For this review, take the finished solid that the model builds, in its own axes (mm). Round coordinates to 2 decimals unless told otherwise and drop trailing zeros. Order: outer loops, then holes, each group sorted by start corner. A loop starts at its lowest first (then second) coordinate and runs counter-clockwise, first axis right, second up. Notation, with made-up numbers: (-6, 69) -> (8, 69) arc R10 cw to (8, 82) -> close; hole circle Ø4 at (-24.75, -28). An arc over 180 degrees is marked (long way). Use a Markdown table: item, result. Add a question column.
1) Consider section B-B (y = 93). State the section outline as (x, z) points (1 decimal).
2) Clearance check with flat-ended pins moving along their axes: P1, Ø10, axis at x = -6, y = 41.5, coming from the -Z side; P2, Ø1.5, axis at x = 0, y = 47.5, coming from the -Z side; P3, Ø1.9, axis at x = 0.5, z = -11, coming from the +Y side. State where each tip first meets the part, or that it passes through.
3) Wall thickness on line 1 along Y through (x, z) = (-1, -10); line 2 along X through (y, z) = (31.5, -0.25): over which ranges is each line inside the solid? List them lowest first. Write a range as [from, to].
4) Consider section C-C (y = 59). State the section outline as (x, z) points.
5) Consider section A-A (x = 0). State the section outline as (y, z) points.
6) Consider section D-D (z = -3.25). State the section outline as (x, y) points, plus the area to 3 significant figures.
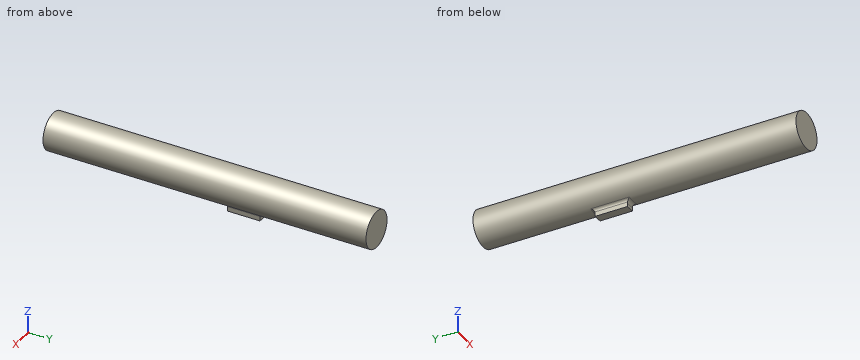
```python
from build123d import *

# Parameters (mm, degrees)
SKETCH1_R           = 8.5
BOSS_EXTRUDE1_DEPTH = 150
SKETCH5_W           = 4
SKETCH5_H           = 11.5
BOSS_EXTRUDE2_DEPTH = 15
FILLET1_R           = 1.5


with BuildPart() as part:
    # Sketch1 → Boss-Extrude1 (new body)
    with BuildSketch(Plane(origin=(0, 0, 0), x_dir=(1, 0, 0), z_dir=(0, 1, 0))):
        Circle(SKETCH1_R)
    extrude(amount=BOSS_EXTRUDE1_DEPTH)

    # Sketch5 → Boss-Extrude2 (add)
    with BuildSketch(Plane(origin=(0, 82.02, 0), x_dir=(1, 0, 0), z_dir=(0, 1, 0))):
        with Locations((0, 5.75)):
            Rectangle(SKETCH5_W, SKETCH5_H)
    extrude(amount=BOSS_EXTRUDE2_DEPTH)

    # Fillet1
    fillet1_edges = [part.edges().sort_by_distance(p)[0] for p in [
        (0, 82.02, -8.5),
        (-2, 89.52, -8.261355821),
        (2, 89.52, -8.261355821),
        (0, 97.02, -8.5),
    ]]
    fillet(fillet1_edges, radius=FILLET1_R)


solid = part.part
```
Results list:
| question | item | result |
|---|---|---|
| 1 | outline | (-3, -8) arc R1.5 cw to (-2, -9.4) -> (-2, -11.5) -> (2, -11.5) -> (2, -9.4) arc R1.5 cw to (3, -8) arc R8.5 ccw (long way) to start |
| 2 | P1 | z = -8.44 |
| 2 | P2 | z = -8.5 |
| 2 | P3 | y = 97.02 |
| 3 | line 1 | [82.02, 97.02] |
| 3 | line 2 | [-8.5, 8.5] |
| 4 | outline | circle Ø17 at (0, 0) |
| 5 | outline | (0, -8.5) -> (80.52, -8.5) arc R1.5 cw to (82.02, -10) -> (82.02, -11.5) -> (97.02, -11.5) -> (97.02, -10) arc R1.5 cw to (98.52, -8.5) -> (150, -8.5) -> (150, 8.5) -> (0, 8.5) -> close |
| 6 | outline | (-7.85, 0) -> (7.85, 0) -> (7.85, 150) -> (-7.85, 150) -> close |
| 6 | area | 2,360 mm2 |
